The model under review builds one solid part; all positions refer to its coordinate system, in mm. A direction names the side the tool comes from. Coordinates: 2 decimals unless noted, no trailing zeros. Order: outer loops, then holes, each group sorted by start corner. A loop starts at its lowest first (then second) coordinate and runs counter-clockwise, first axis right, second up. Notation, with made-up numbers: (-17, 31) -> (30, 31) arc R29 cw to (30, 60) -> close; hole circle Ø7 at (-32, 29.25). An arc over 180 degrees is marked (long way). Use one line per item in the form item = value.
from build123d import *

# Parameters (mm, degrees)
SKETCH1_W           = 68.987924
SKETCH1_H           = 80.264
BOSS_EXTRUDE3_DEPTH = 2.54
BOSS_EXTRUDE4_DEPTH = 31.75
SKETCH1_6_W         = 46.99
SKETCH1_6_H         = 2.54
BOSS_EXTRUDE5_DEPTH = 13.462
SKETCH2_W           = 2.54
SKETCH2_H           = 31.75
BOSS_EXTRUDE6_DEPTH = 34.29
BOSS_EXTRUDE7_DEPTH = 31.75


with BuildPart() as part:
    # Sketch1 → Boss-Extrude3 (new body)
    with BuildSketch(Plane(origin=(0, 0, 0), x_dir=(0, 0, -1), z_dir=(1, 0, 0))):
        with Locations((0.050038, -1.397)):
            Rectangle(SKETCH1_W, SKETCH1_H)
    extrude(amount=BOSS_EXTRUDE3_DEPTH)

    # Sketch1<5> → Boss-Extrude4 (add)
    with BuildSketch(Plane(origin=(0, 0, 0), x_dir=(0, 0, -1), z_dir=(1, 0, 0))):
        Polygon((34.544, 38.735), (32.004, 38.735), (32.004, 36.195), (32.004, -38.989), (-31.903924, -38.989), (-31.903924, 38.735), (-34.443924, 38.735), (-34.443924, 32.385), (-34.443924, -41.529), (34.544, -41.529), align=None)
    extrude(amount=-BOSS_EXTRUDE4_DEPTH)

    # Sketch1<6> → Boss-Extrude5 (add)
    with BuildSketch(Plane(origin=(0, 0, 0), x_dir=(0, 0, -1), z_dir=(1, 0, 0))):
        with Locations((8.509, 37.465)):
            Rectangle(SKETCH1_6_W, SKETCH1_6_H)
    extrude(amount=-BOSS_EXTRUDE5_DEPTH)

    # Sketch2 → Boss-Extrude6 (add)
    with BuildSketch(Plane.ZY):
        with Locations((17.526, -16.764)):
            Rectangle(SKETCH2_W, SKETCH2_H)
    extrude(amount=BOSS_EXTRUDE6_DEPTH)

    # Sketch3 → Boss-Extrude7 (add)
    with BuildSketch(Plane.XZ.offset(32.639)):
        with BuildLine():
            Line((-34.29, 18.796), (-40.086328026, 18.796))
            ThreePointArc((-40.086328026, 18.796), (-40.695965663, 18.338670907), (-40.427477229, 17.625423468))
            Line((-40.427477229, 17.625423468), (-34.29, 13.716))
            Line((-34.29, 13.716), (-34.29, 18.796))
        make_face()
    extrude(amount=-BOSS_EXTRUDE7_DEPTH)


solid = part.part
Item 1: We need section C-C (x = -5). Write out the cut boundary in (y, z) (3 decimals), plus the area to 3 significant figures.
Results found:
outline = (-41.529, -34.544) -> (38.735, -34.544) -> (38.735, 14.986) -> (36.195, 14.986) -> (36.195, -32.004) -> (-38.989, -32.004) -> (-38.989, 31.904) -> (38.735, 31.904) -> (38.735, 34.444) -> (-41.529, 34.444) -> close; (-32.639, 16.256) -> (-0.889, 16.256) -> (-0.889, 18.796) -> (-32.639, 18.796) -> close
area = 770 mm²
Item 2: Draft analysis for pull direction Y (two halves, no side actions). For faces 6 (the face through (-16, 0, -32.004)), 7 (the face through (-16, -38.989, 0)), 8 (the face through (-14, -41.529, 0)), 9 (the face through (-7, 37, 14.986)), state which applies: released by +Y, released by -Y, zero draft, split by the parting line, or undercut.
Results found:
face_6 = undercut
face_7 = undercut
face_8 = released by -Y
face_9 = zero draft
Item 3: We need section B-B (y = 29). Write out the cut boundary in (x, z), plus the area to 3 significant figures.
Results found:
outline = (-31.75, -34.54) -> (2.54, -34.54) -> (2.54, 34.44) -> (-31.75, 34.44) -> (-31.75, 31.9) -> (0, 31.9) -> (0, -32) -> (-31.75, -32) -> close
area = 337 mm²
Item 4: Tool access review of faces 1 (the face through (-17, -17, 16.256)), 2 (the face through (-34.29, -17, 15)), 3 (the face through (-14, -2, -34.544)), 4 (the face through (-21, -0.889, 17)), 5 (the face through (-7, 36.195, -8)): name each direction out of +Z, -Z, +X, -X, +Y, -Y from which nothing blocks a thin tool from reaching the whole face with its end or side.
Results found:
face_1 = +Y
face_2 = -Z, +Y, -Y
face_3 = -Z, +X, -X, +Y, -Y
face_4 = -X, +Y
face_5 = -X
Item 5: To check wall thickness, follow L1, parallel to Z at x = -4.5, y = -31; L2, parallel to Y at x = -2, z = -9.5 (3 decimals); L3, parallel to Z at x = -2.5, y = 22.5. State the ranges of each line that lie inside material, in increasing order. Write a range as from..to.
Results found:
L1 = -34.54..-32, 16.26..18.8, 31.9..34.44
L2 = -41.529..-38.989, 36.195..38.735
L3 = -34.54..-32, 31.9..34.44
Item 6: Clearance check with flat-ended pins moving along their axes: pin 1 (1.5 mm diameter, centred on y = -3.5, z = -22.5, fed in from -X); pin 2 (6 mm diameter, centred on x = -28.5, z = -13, fed in from +Y); pin 3 (1.5 mm diameter, centred on x = -13.5, z = 17, fed in from +Y). State where each tip first meets the part, or that it passes through.
Results found:
pin_1 = 0
pin_2 = -38.99
pin_3 = -0.89
Item 7: We need section A-A (x = -28). Write out the cut boundary in (y, z) (3 decimals).
Results found:
outline = (-41.529, -34.544) -> (38.735, -34.544) -> (38.735, -32.004) -> (-38.989, -32.004) -> (-38.989, 31.904) -> (38.735, 31.904) -> (38.735, 34.444) -> (-41.529, 34.444) -> close; (-32.639, 16.256) -> (-0.889, 16.256) -> (-0.889, 18.796) -> (-32.639, 18.796) -> close
Item 8: We need section D-D (z = -23). Write out the cut boundary in (x, y) (3 decimals).
Results found:
outline = (-31.75, -41.529) -> (2.54, -41.529) -> (2.54, 38.735) -> (-13.462, 38.735) -> (-13.462, 36.195) -> (0, 36.195) -> (0, -38.989) -> (-31.75, -38.989) -> close
